Source: CAD feature listing. Evaluate the final solid. Frame: model axes, mm. A direction names the side the tool comes from. Round coordinates to 2 decimals unless told otherwise and drop trailing zeros. Loops run counter-clockwise (first coordinate to the right, second up) from the corner with the lowest first, then second, coordinate; pieces in that order, holes last. Notation, with made-up numbers: M 17.5,87.5 L 25.5,87.5 A25 ccw 25.5,107.5 Z; hole C 45.5,60 d3. An arc over 180 degrees is marked long. Write each question's results on one line, items separated by ' | '. Start each with the question number.
1. Ray query, line 1 (Y direction, x = 54.75, z = -9.45); line 2 (Y direction, x = 55.25, z = -13.5); line 3 (Z direction, x = 52.5, y = -0.5). Return the intervals inside material, ascending.
2. Section C-C on z = -22. Output: boundary loops of the cut face in (x, y).
3. Section B-B on x = 49. Output: boundary loops of the cut face in (y, z) (3 decimals), and give its area (3 significant figures).
4. Section A-A on y = 0. Output: boundary loops of the cut face in (x, z).
5. Contact query for flat-ended pins moving along their axis: pin 1 Ø2 at (x, z) = (52, -11) entering from +Y; pin 2 Ø5.5 at (y, z) = (-5.5, -12) entering from +X; pin 3 Ø4 at (x, z) = (52.5, -21) entering from -Y; pin 4 Ø1 at (x, y) = (44.5, -10.5) entering from -Z. Output: stop coordinate, or through.
6. Draft query along Y for faces 1 (the cylindrical face through (54.59, 0.04, -7.45)), 2 (the flat face through (49, -19, -8)), 3 (the cylindrical face through (44, 0, -18)), 4 (the flat face through (55.6, 0, -15)). Return one class per face: released by +Y, released by -Y, zero draft, split by the parting line, or undercut.
7. Set-up query: faces 5 (the flat face through (49, 19, -3)), 6 (the cylindrical face through (54.586, 14.545, -8.8)), 7 (the flat face through (44.6, -3, -18)). Return all of +Z, -Z, +X, -X, +Y, -Y with unobstructed straight access to the full face (end or side cutting, diameter ignored); none if empty.
from build123d import *

# Parameters (mm, degrees)
BOSS_EXTRU_1_DEPTH           = 114
ESQUISSE2_R                  = 22.55
ENL_V_MAT_EXTRU_2_DEPTH      = 5
ENL_V_START                  = -5
ESQUISSE4_R                  = 22.55
ENL_V_MAT_EXTRU_3_DEPTH      = 5
ESQUISSE5_R                  = 1
ENL_V_MAT_EXTRU_4_DEPTH      = 118.883477756
BOSS_EXTRU_2_START           = -2
BOSS_EXTRU_2_DEPTH           = 2
BOSS_EXTRU_3_START           = 9
BOSS_EXTRU_3_DEPTH           = 9
BOSS_EXTRU_4_START           = 2
BOSS_EXTRU_4_DEPTH           = 2
BOSS_EXTRU_5_START           = -2
BOSS_EXTRU_5_DEPTH           = 2
BOSS_EXTRU_6_START           = 9
BOSS_EXTRU_6_DEPTH           = 9
BOSS_EXTRU_7_START           = 2
BOSS_EXTRU_7_DEPTH           = 2
ESQUISSE12_W                 = 13.751826503
ESQUISSE12_H                 = 1
ESQUISSE12_W_2               = 11.167500513
ENL_V_MAT_EXTRU_5_DEPTH      = 95.05366831
BOSS_EXTRU_8_START           = -13
BOSS_EXTRU_8_DEPTH           = 13
BOSS_EXTRU_9_START           = -13
BOSS_EXTRU_9_DEPTH           = 13
ENL_V_MAT_EXTRU_6_DEPTH      = 94.846110875
ENL_V_MAT_EXTRU_7_DEPTH      = 119.048305907
ENL_V_MAT_EXTRU_7_DEPTH_BACK = 119.048305907
ESQUISSE16_R                 = 2
ENL_V_MAT_EXTRU_8_DEPTH      = 119.048305907
ENL_V_MAT_EXTRU_8_DEPTH_BACK = 119.048305907
ESQUISSE17_W                 = 59.614758746
ESQUISSE17_H                 = 46.78428057
ESQUISSE17_W_2               = 63.060495968
ESQUISSE17_H_2               = 47.274864603
BOSS_EXTRU_10_START          = -2
ESQUISSE18_R                 = 0.95
BOSS_EXTRU_10_DEPTH          = 2


with BuildPart() as part:
    # Esquisse1 → Boss.-Extru.1 (new body)
    with BuildSketch(Plane(origin=(0, 0, 0), x_dir=(0, 0, -1), z_dir=(1, 0, 0))):
        with BuildLine():
            Line((14.144270925, 14.14), (17.975320492, 17.947474134))
            ThreePointArc((17.975320492, 17.947474134), (24.05, 0), (17.975320492, -17.947474134))
            Line((17.975320492, -17.947474134), (14.144270925, -14.14))
            ThreePointArc((14.144270925, -14.14), (20, 0), (14.144270925, 14.14))
        make_face()
    extrude(amount=BOSS_EXTRU_1_DEPTH)

    # Esquisse2 → Enlèv. mat.-Extru.2 (cut)
    with BuildSketch(Plane.ZY):
        Circle(ESQUISSE2_R)
    extrude(amount=-ENL_V_MAT_EXTRU_2_DEPTH, mode=Mode.SUBTRACT)

    # Esquisse4 → Enlèv. mat.-Extru.3 (cut)
    with BuildSketch(Plane(origin=(114, 0, 0), x_dir=(0, 0, -1), z_dir=(1, 0, 0)).offset(ENL_V_START)):
        Circle(ESQUISSE4_R)
    extrude(amount=ENL_V_MAT_EXTRU_3_DEPTH, mode=Mode.SUBTRACT)

    # Esquisse5 → Enlèv. mat.-Extru.4 (cut, through all)
    with BuildSketch(Plane.XY):
        with Locations((2.5, 0)):
            Circle(ESQUISSE5_R)
        with Locations((111.5, 0)):
            Circle(ESQUISSE5_R)
    extrude(amount=-ENL_V_MAT_EXTRU_4_DEPTH, mode=Mode.SUBTRACT)

    # Esquisse6 → Boss.-Extru.2 (add)
    with BuildSketch(Plane(origin=(88.7, 0, 0), x_dir=(0, 0, -1), z_dir=(1, 0, 0)).offset(BOSS_EXTRU_2_START)):
        with BuildLine():
            Line((0, 17), (0, 20))
            ThreePointArc((0, 20), (20, 0), (0, -20))
            Line((0, -20), (0, -17))
            ThreePointArc((0, -17), (17, 0), (0, 17))
        make_face()
    extrude(amount=BOSS_EXTRU_2_DEPTH)

    # Esquisse7 → Boss.-Extru.3 (add)
    with BuildSketch(Plane.ZY.offset(-86.7).offset(BOSS_EXTRU_3_START)):
        with BuildLine():
            Line((0, 20), (0, 19))
            ThreePointArc((0, 19), (-19, 0), (0, -19))
            Line((0, -19), (0, -20))
            ThreePointArc((0, -20), (-20, 0), (0, 20))
        make_face()
    extrude(amount=-BOSS_EXTRU_3_DEPTH)

    # Esquisse8 → Boss.-Extru.4 (add)
    with BuildSketch(Plane.ZY.offset(-77.7).offset(BOSS_EXTRU_4_START)):
        with BuildLine():
            Line((0, 20), (0, 18))
            ThreePointArc((0, 18), (-18, 0), (0, -18))
            Line((0, -18), (0, -20))
            ThreePointArc((0, -20), (-20, 0), (0, 20))
        make_face()
    extrude(amount=-BOSS_EXTRU_4_DEPTH)

    # Esquisse9 → Boss.-Extru.5 (add)
    with BuildSketch(Plane(origin=(55.6, 0, 0), x_dir=(0, 0, -1), z_dir=(1, 0, 0)).offset(BOSS_EXTRU_5_START)):
        with BuildLine():
            Line((0, 20), (0, 17))
            ThreePointArc((0, 17), (17, 0), (0, -17))
            Line((0, -17), (0, -20))
            ThreePointArc((0, -20), (20, 0), (0, 20))
        make_face()
    extrude(amount=BOSS_EXTRU_5_DEPTH)

    # Esquisse10 → Boss.-Extru.6 (add)
    with BuildSketch(Plane.ZY.offset(-53.6).offset(BOSS_EXTRU_6_START)):
        with BuildLine():
            Line((0, 20), (0, 19))
            ThreePointArc((0, 19), (-19, 0), (0, -19))
            Line((0, -19), (0, -20))
            ThreePointArc((0, -20), (-20, 0), (0, 20))
        make_face()
    extrude(amount=-BOSS_EXTRU_6_DEPTH)

    # Esquisse11 → Boss.-Extru.7 (add)
    with BuildSketch(Plane.ZY.offset(-44.6).offset(BOSS_EXTRU_7_START)):
        with BuildLine():
            Line((0, 20), (0, 18))
            ThreePointArc((0, 18), (-18, 0), (0, -18))
            Line((0, -18), (0, -20))
            ThreePointArc((0, -20), (-20, 0), (0, 20))
        make_face()
    extrude(amount=-BOSS_EXTRU_7_DEPTH)

    # Esquisse12 → Enlèv. mat.-Extru.5 (cut, through all)
    with BuildSketch(Plane(origin=(88.7, 0, 0), x_dir=(0, 0, -1), z_dir=(1, 0, 0))):
        with Locations((6.875913252, -19.5)):
            Rectangle(ESQUISSE12_W, ESQUISSE12_H)
        with Locations((5.583750257, 19.5)):
            Rectangle(ESQUISSE12_W_2, ESQUISSE12_H)
    extrude(amount=-ENL_V_MAT_EXTRU_5_DEPTH, mode=Mode.SUBTRACT)

    # Esquisse13 → Boss.-Extru.8 (add)
    with BuildSketch(Plane(origin=(88.7, 0, 0), x_dir=(0, 0, -1), z_dir=(1, 0, 0)).offset(BOSS_EXTRU_8_START)):
        with BuildLine():
            Line((17.975320492, 17.947474134), (14.144270925, 14.14))
            ThreePointArc((14.144270925, 14.14), (10.480241973, 17.034216395), (6.244997998, 19))
            Line((6.244997998, 19), (17.4396757, 18.627232183))
            ThreePointArc((17.4396757, 18.627232183), (17.709986765, 18.289314213), (17.975320492, 17.947474134))
        make_face()
        with BuildLine():
            Line((14.144270925, -14.14), (17.975320492, -17.947474134))
            ThreePointArc((17.975320492, -17.947474134), (17.559611782, -18.478549847), (17.131891216, -19))
            Line((17.131891216, -19), (6.244997998, -19))
            ThreePointArc((6.244997998, -19), (10.480241973, -17.034216395), (14.144270925, -14.14))
        make_face()
    extrude(amount=BOSS_EXTRU_8_DEPTH)

    # Esquisse14 → Boss.-Extru.9 (add)
    with BuildSketch(Plane(origin=(55.6, 0, 0), x_dir=(0, 0, -1), z_dir=(1, 0, 0)).offset(BOSS_EXTRU_9_START)):
        with BuildLine():
            Line((14.144270925, 14.14), (17.975320492, 17.947474134))
            ThreePointArc((17.975320492, 17.947474134), (17.709986765, 18.289314213), (17.4396757, 18.627232183))
            Line((17.4396757, 18.627232183), (6.244997998, 19))
            ThreePointArc((6.244997998, 19), (10.480241973, 17.034216395), (14.144270925, 14.14))
        make_face()
        with BuildLine():
            Line((14.144270925, -14.14), (17.975320492, -17.947474134))
            ThreePointArc((17.975320492, -17.947474134), (17.559611782, -18.478549847), (17.131891216, -19))
            Line((17.131891216, -19), (6.244997998, -19))
            ThreePointArc((6.244997998, -19), (10.480241973, -17.034216395), (14.144270925, -14.14))
        make_face()
    extrude(amount=BOSS_EXTRU_9_DEPTH)

    # Esquisse15 → Enlèv. mat.-Extru.6 (cut, through all)
    with BuildSketch(Plane(origin=(88.7, 0, 0), x_dir=(0, 0, -1), z_dir=(1, 0, 0))):
        with BuildLine():
            Line((14.409304815, 20.298729325), (16.901493379, 24.760797344))
            Line((16.901493379, 24.760797344), (24.890475951, 20.298729325))
            Line((24.890475951, 20.298729325), (20.895984665, 15.394026057))
            ThreePointArc((20.895984665, 15.394026057), (17.822174246, 18.070587713), (14.409304815, 20.298729325))
        make_face()
        with BuildLine():
            Line((14.409304815, -20.298729325), (16.901493379, -24.760797344))
            Line((16.901493379, -24.760797344), (22.934233847, -18.464332541))
            Line((22.934233847, -18.464332541), (20.431131458, -15.848802481))
            ThreePointArc((20.431131458, -15.848802481), (17.561732891, -18.265269573), (14.409304815, -20.298729325))
        make_face()
    extrude(amount=-ENL_V_MAT_EXTRU_6_DEPTH, mode=Mode.SUBTRACT)

    # Esquisse16 → Enlèv. mat.-Extru.7 (cut, two sides: drawn at the far end of the back side and taken through both)
    with BuildSketch(Plane.XY.offset(-ENL_V_MAT_EXTRU_7_DEPTH_BACK)):
        with Locations((114, 13)):
            Circle(ESQUISSE16_R)
        with Locations((114, -13)):
            Circle(ESQUISSE16_R)
    extrude(amount=ENL_V_MAT_EXTRU_7_DEPTH + ENL_V_MAT_EXTRU_7_DEPTH_BACK, mode=Mode.SUBTRACT)

    # Esquisse17 → Enlèv. mat.-Extru.8 (cut, two sides: drawn at the far end of the back side and taken through both)
    with BuildSketch(Plane.XY.offset(-ENL_V_MAT_EXTRU_8_DEPTH_BACK)):
        with Locations((12.792620627, -4.392140285)):
            Rectangle(ESQUISSE17_W, ESQUISSE17_H)
        with Locations((87.130247984, -4.637432302)):
            Rectangle(ESQUISSE17_W_2, ESQUISSE17_H_2)
    extrude(amount=ENL_V_MAT_EXTRU_8_DEPTH + ENL_V_MAT_EXTRU_8_DEPTH_BACK, mode=Mode.SUBTRACT)

    # Esquisse18 → Boss.-Extru.10 (add)
    with BuildSketch(Plane(origin=(55.6, 0, 0), x_dir=(0, 0, -1), z_dir=(1, 0, 0)).offset(BOSS_EXTRU_10_START)):
        with BuildLine():
            ThreePointArc((9.45, 2), (7.45, 0), (9.45, -2))
            add(Edge.make_bspline(
                [(9.45, -2), (14.286652035, -1.165113332), (15.178639222, -7.655645719)],
                knots=[0, 0, 0, 1, 1, 1], degree=2))
            ThreePointArc((15.178639222, -7.655645719), (17, 0), (15.178639222, 7.655645719))
            add(Edge.make_bspline(
                [(9.45, 2), (14.286652035, 1.165113332), (15.178639222, 7.655645719)],
                knots=[0, 0, 0, 1, 1, 1], degree=2))
        make_face()
        with Locations((9.45, 0)):
            Circle(ESQUISSE18_R, mode=Mode.SUBTRACT)
    extrude(amount=BOSS_EXTRU_10_DEPTH)


solid = part.part
Taken from the geometry:
1) line 1: -19 to -14.13, -2 to -0.95, 0.95 to 2, 14.13 to 18.89 | line 2: -19 to -10.33, -3.21 to 3.21, 10.33 to 18.76 | line 3: -24.05 to -18.99
2) outline: M 42.6,-10.81 L 55.6,-10.81 L 55.6,10.81 L 42.6,10.81 Z
3) outline: M -19,-16.521 A29.55 ccw -17.963,-17.963 A29.55 ccw -17.947,-17.975 A29.55 ccw 17.947,-17.975 A29.55 ccw 17.963,-17.963 A29.55 ccw 18.64,-17.042 L 19,-6.245 L 19,0 A19 cw -19,0 Z | area: 261 mm^2
4) outline: M 42.6,-24.05 L 55.6,-24.05 L 55.6,-10.4 L 53.6,-10.4 L 53.6,-19 L 44.6,-19 L 44.6,-18 L 42.6,-18 Z; M 53.6,-8.5 L 55.6,-8.5 L 55.6,-7.45 L 53.6,-7.45 Z
5) pin 1: y = 18.87 | pin 2: x = 55.6 | pin 3: y = -16.52 | pin 4: z = -22.31
6) face 1: undercut | face 2: released by -Y | face 3: undercut | face 4: zero draft
7) face 5: +Z, -Z, +X, -X, +Y | face 6: +Z, +X, -X | face 7: +Z
